```python
from build123d import *

# Parameters (mm, degrees)
SKETCH_W     = 5.8
SKETCH_H     = 2.95
PAD_DEPTH    = 2.25
SKETCH001_W  = 5
SKETCH001_H  = 2.5
PAD001_DEPTH = 3.975
FILLET_R     = 2.99
CHAMFER_SIZE = 2.9999
FILLET001_R  = 3
FILLET002_R  = 1


with BuildPart() as part:
    # Sketch → Pad (new body)
    with BuildSketch(Plane.YZ):
        with BuildLine():
            Line((-6.875, -15.125), (6.875, -15.125))
            Line((6.875, -15.125), (6.875, 15.125))
            Line((6.875, 15.125), (-6.875, 15.125))
            Line((-6.875, 15.125), (-6.875, 2.25))
            ThreePointArc((-6.875, 2.25), (-3.300315, 1.928152), (0.277037, 2.218873))
            ThreePointArc((0.277037, -2.218873), (2.9, 0), (0.277037, 2.218873))
            ThreePointArc((0.277037, -2.218873), (-3.300315, -1.928152), (-6.875, -2.25))
            Line((-6.875, -2.25), (-6.875, -15.125))
        make_face()
        with Locations((0, 11.275)):
            Rectangle(SKETCH_W, SKETCH_H, mode=Mode.SUBTRACT)
        with Locations((0, -11.275)):
            Rectangle(SKETCH_W, SKETCH_H, mode=Mode.SUBTRACT)
    extrude(amount=-PAD_DEPTH)

    # Sketch001 (on DatumPlane) → Pad001 (join)
    with BuildSketch(Plane.ZX.offset(6.875)):
        with BuildLine():
            Line((-6, 0), (15.125, 0))
            Line((15.125, 0), (18.125, 0))
            Line((18.125, 0), (18.125, 16.606602))
            Line((18.125, 16.606602), (15.125, 16.606602))
            Line((2.303301, 16.606602), (15.125, 16.606602))
            ThreePointArc((2.303301, 16.606602), (-3.568019, 14.174621), (-6, 8.303301))
            Line((-6, 0), (-6, 8.303301))
        make_face()
        with Locations((12.625, 4.553301)):
            Rectangle(SKETCH001_W, SKETCH001_H, mode=Mode.SUBTRACT)
        with Locations((12.625, 12.053301)):
            Rectangle(SKETCH001_W, SKETCH001_H, mode=Mode.SUBTRACT)
        Polygon((4.267767, 0.5), (7.803301, 4.035534), (6.035534, 5.803301), (2.5, 2.267767), align=None, mode=Mode.SUBTRACT)
        Polygon((-1.035534, 5.803301), (2.5, 9.338835), (0.732233, 11.106602), (-2.803301, 7.571068), align=None, mode=Mode.SUBTRACT)
    extrude(amount=-PAD001_DEPTH)

    # Fillet
    fillet_edges = [part.edges().sort_by_distance(p)[0] for p in [
        (0, 4.8875, -6),
        (16.606602, 4.8875, 18.125),
    ]]
    fillet(fillet_edges, radius=FILLET_R)

    # Chamfer
    chamfer_edges = [part.edges().sort_by_distance(p)[0] for p in [
        (0, 4.8875, 18.125),
    ]]
    chamfer(chamfer_edges, length=CHAMFER_SIZE)

    # Fillet001
    fillet001_edges = [part.edges().sort_by_distance(p)[0] for p in [
        (2.9999, 4.8875, 18.125),
    ]]
    fillet(fillet001_edges, radius=FILLET001_R)

    # Fillet002
    fillet002_edges = [part.edges().sort_by_distance(p)[0] for p in [
        (-1.125, -6.875, 2.25),
        (-1.125, -6.875, -2.25),
    ]]
    fillet(fillet002_edges, radius=FILLET002_R)


solid = part.part
```
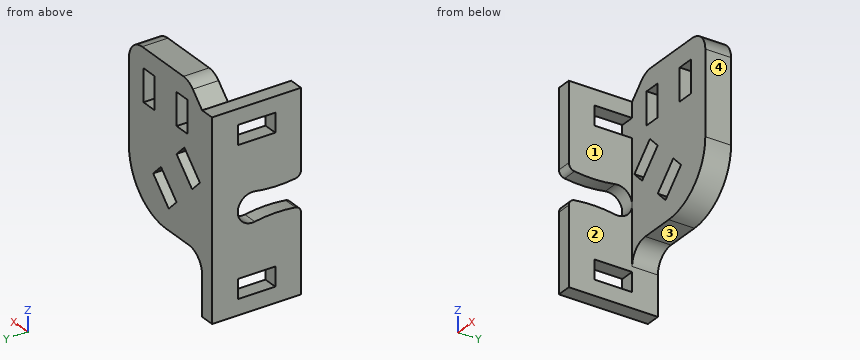
The model under review builds one solid part; all positions refer to its coordinate system, in mm. Face numbers are marked on the shaded views. A direction names the side the tool comes from. Round coordinates to 2 decimals unless told otherwise and drop trailing zeros. Order: outer loops, then holes, each group sorted by start corner. A loop starts at its lowest first (then second) coordinate and runs counter-clockwise, first axis right, second up. Notation, with made-up numbers: (84, -5.5) -> (143, -5.5) arc R27 cw to (143, 26.5) -> close; hole circle Ø4 at (-26, 54). An arc over 180 degrees is marked (long way). Use a Markdown table: item, result.
Q1. Tool access review of the marked faces 1, 2, 3 and 4: name each direction out of +Z, -Z, +X, -X, +Y, -Y from which nothing blocks a thin tool from reaching the whole face with its end or side.
Values:
| item | result |
|---|---|
| face 1 | +Z, -Z, +X, -Y |
| face 2 | -Z, +X, -Y |
| face 3 | -Z, +X, +Y, -Y |
| face 4 | +Z, -Z, +X, +Y, -Y |
Q2. We need section A-A on z = 13.5. Write out the cut boundary in (x, y) (3 decimals), then the cut area to 3 significant figures.
Values:
| item | result |
|---|---|
| outline | (-2.25, -6.875) -> (0, -6.875) -> (0, 2.9) -> (3.303, 2.9) -> (3.303, 6.875) -> (-2.25, 6.875) -> close; (5.803, 2.9) -> (10.803, 2.9) -> (10.803, 6.875) -> (5.803, 6.875) -> close; (13.303, 2.9) -> (16.607, 2.9) -> (16.607, 6.875) -> (13.303, 6.875) -> close |
| area | 77.1 mm^2 |
Q3. Clearance check with flat-ended pins moving along their axes: P1, Ø5, axis at y = -1.5, z = 11, coming from the +X side; P2, Ø8, axis at x = 0.5, y = 0, coming from the -Z side (3 decimals); P3, Ø6, axis at y = 0.65, z = 0, coming from the +X side; P4, Ø1.2, axis at x = 5.5, y = 4.5, coming from the -Z side. State where each tip first meets the part, or that it passes through.
Values:
| item | result |
|---|---|
| P1 | stops at x = 0 |
| P2 | stops at z = -15.125 |
| P3 | stops at x = 16.6 |
| P4 | stops at z = -6 |
Q4. We need section B-B on y = 0.65. Write out the cut boundary in (x, z) (3 decimals).
Values:
| item | result |
|---|---|
| outline | (-2.25, -15.125) -> (0, -15.125) -> (0, -12.75) -> (-2.25, -12.75) -> close; (-2.25, -9.8) -> (0, -9.8) -> (0, -2.25) -> (-2.25, -2.25) -> close; (-2.25, 2.25) -> (0, 2.25) -> (0, 9.8) -> (-2.25, 9.8) -> close; (-2.25, 12.75) -> (0, 12.75) -> (0, 15.125) -> (-2.25, 15.125) -> close |
Q5. For line 1 (Z direction, x = -0.95, y = 0.65) (3 decimals); line 2 (Z direction, x = 5.5, y = 4.25) (3 decimals); line 3 (Y direction, x = 2.25, z = 12) (3 decimals), list the stretches that pass through material, from the lowest coordinate up.
Values:
| item | result |
|---|---|
| line 1 | z = -15.125 to -12.75, -9.8 to -2.25, 2.25 to 9.8, 12.75 to 15.125 |
| line 2 | z = -6 to 5.732, 6.339 to 10.125, 15.125 to 18.125 |
| line 3 | y = 2.9 to 6.875 |
Q6. We need section C-C on z = -11. Write out the cut boundary in (x, y) (3 decimals), then the cut area to 3 significant figures.
Values:
| item | result |
|---|---|
| outline | (-2.25, -6.875) -> (0, -6.875) -> (0, -2.9) -> (-2.25, -2.9) -> close; (-2.25, 2.9) -> (0, 2.9) -> (0, 6.875) -> (-2.25, 6.875) -> close |
| area | 17.9 mm^2 |
Q7. We need section D-D on x = 12.5. Write out the cut boundary in (y, z) (3 decimals), then the cut area to 3 significant figures.
Values:
| item | result |
|---|---|
| outline | (2.9, -4.861) -> (6.875, -4.861) -> (6.875, 10.125) -> (2.9, 10.125) -> close; (2.9, 15.125) -> (6.875, 15.125) -> (6.875, 18.125) -> (2.9, 18.125) -> close |
| area | 71.5 mm^2 |
